Here's how the part is built. I have some questions about the finished solid (model axes, mm). Face numbers are marked on the shaded views. A direction names the side the tool comes from. Give positions to 0.01 mm unless a question says otherwise; leave off trailing zeros. Loops run counter-clockwise (first coordinate to the right, second up) from the corner with the lowest first, then second, coordinate; pieces in that order, holes last. Notation, with made-up numbers: (67.5, -30.5) - (125.5, -30.5) arc R23 cw to (125.5, -11.5) - close; hole circle Ø8 at (63.5, 52). An arc over 180 degrees is marked (long way). Use a Markdown table: item, result.
from build123d import *

# Parameters (mm, degrees)
CUT_EXTRUDE1_DEPTH       = 91
CUT_EXTRUDE13_START      = 79.372539
SKETCH35_W               = 20
SKETCH35_H               = 8.35
CUT_EXTRUDE13_DEPTH      = 10.627461
CIRPATTERN1_COUNT        = 2
CUT_EXTRUDE14_DEPTH      = 64
SKETCH38_W               = 301.896550135
SKETCH38_H               = 232.512752758
CUT_EXTRUDE15_DEPTH      = 13
SKETCH39_W               = 54.010562882
SKETCH39_H               = 10
SKETCH39_W_2             = 56.106077308
BOSS_EXTRUDE1_DEPTH      = 10
SKETCH17_R               = 5.5
CUT_EXTRUDE18_DEPTH      = 181
CUT_EXTRUDE18_DEPTH_BACK = 1
SKETCH42_R               = 15.875
CUT_EXTRUDE19_DEPTH      = 40


with BuildPart() as part:
    # Sketch3 → Revolve2 (revolve)
    with BuildSketch(Plane(origin=(0, 0, 0), x_dir=(0, 0, -1), z_dir=(1, 0, 0))):
        Polygon((-45, 80), (0, 80), (0, 90), (-63, 90), (-63, 15), (-45, 15), (-45, 27.5), (-47.5, 27.5), (-47.5, 73), (-45, 73), align=None)
    revolve(axis=Axis((0, 0, 0), (0, 0, 1)))

    # Sketch4 → Cut-Extrude1 (cut, through all)
    with BuildSketch(Plane(origin=(0, 0, 0), x_dir=(1, 0, 0), z_dir=(0, 1, 0))):
        Polygon((10, -53), (10, -45), (-10, -45), (-10, -53), (-6, -53), (-6, -60), (-10, -60), (-10, -63), (10, -63), (10, -60), (6, -60), (6, -53), align=None)
    cut_extrude1 = extrude(amount=CUT_EXTRUDE1_DEPTH, mode=Mode.SUBTRACT)

    # Sketch35 → Cut-Extrude13 (cut)
    with BuildSketch(Plane(origin=(0, 0, 0), x_dir=(1, 0, 0), z_dir=(0, 1, 0)).offset(CUT_EXTRUDE13_START)):
        with Locations((0, -40.825)):
            Rectangle(SKETCH35_W, SKETCH35_H)
    cut_extrude13 = extrude(amount=CUT_EXTRUDE13_DEPTH, mode=Mode.SUBTRACT)

    # CirPattern1: Cut-Extrude1, Cut-Extrude13 ×2 about axis
    cirpattern1_axis = Axis((0, 0, 0), (0, 0, 1))
    for i in range(1, CIRPATTERN1_COUNT):
        add(cut_extrude1.rotate(cirpattern1_axis, i * 360 / CIRPATTERN1_COUNT), mode=Mode.SUBTRACT)
        add(cut_extrude13.rotate(cirpattern1_axis, i * 360 / CIRPATTERN1_COUNT), mode=Mode.SUBTRACT)

    # Sketch37 → Cut-Extrude14 (cut, through all)
    with BuildSketch(Plane.XY.offset(63)):
        with BuildLine():
            Line((-28, -66.332495807), (-28, -17.464249197))
            ThreePointArc((-28, -17.464249197), (-33, 0), (-28, 17.464249197))
            Line((-28, 17.464249197), (-28, 66.332495807))
            ThreePointArc((-28, 66.332495807), (-72, 0), (-28, -66.332495807))
        make_face()
        with BuildLine():
            Line((28, -17.464249197), (28, -66.332495807))
            ThreePointArc((28, -66.332495807), (72, 0), (28, 66.332495807))
            Line((28, 66.332495807), (28, 17.464249197))
            ThreePointArc((28, 17.464249197), (33, 0), (28, -17.464249197))
        make_face()
    extrude(amount=-CUT_EXTRUDE14_DEPTH, mode=Mode.SUBTRACT)

    # Sketch38 → Cut-Extrude15 (cut)
    with BuildSketch(Plane(origin=(0, 0, 0), x_dir=(-1, 0, 0), z_dir=(0, 0, -1))):
        with Locations((8.285843347, -5.180042081)):
            Rectangle(SKETCH38_W, SKETCH38_H)
    extrude(amount=-CUT_EXTRUDE15_DEPTH, mode=Mode.SUBTRACT)

    # Sketch39 → Boss-Extrude1 (add)
    with BuildSketch(Plane.XY.offset(63)):
        with Locations((47.183112068, 0)):
            Rectangle(SKETCH39_W, SKETCH39_H)
        with Locations((-51.507331201, 0)):
            Rectangle(SKETCH39_W_2, SKETCH39_H)
    extrude(amount=-BOSS_EXTRUDE1_DEPTH)

    # Sketch17 → Cut-Extrude18 (cut, two sides)
    with BuildSketch(Plane(origin=(-90, 0, 0), x_dir=(0, 0, -1), z_dir=(1, 0, 0))) as cut_extrude18_sk:
        with Locations((-27.5, 0)):
            Circle(SKETCH17_R)
    extrude(amount=CUT_EXTRUDE18_DEPTH, mode=Mode.SUBTRACT)
    extrude(cut_extrude18_sk.sketch, amount=-CUT_EXTRUDE18_DEPTH_BACK, mode=Mode.SUBTRACT)

    # Sketch42 → Cut-Extrude19 (cut)
    with BuildSketch(Plane.XY.offset(63)):
        Circle(SKETCH42_R)
    extrude(amount=-CUT_EXTRUDE19_DEPTH, mode=Mode.SUBTRACT)


solid = part.part
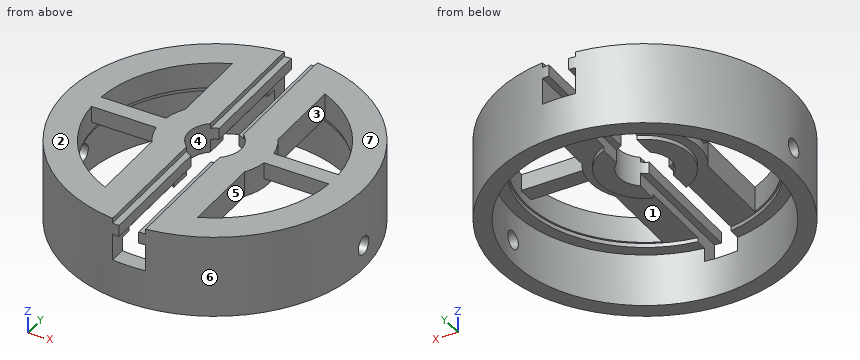
(1) Suppose I cut it at B-B on y = -50.5. Count the separate pieces of the cut face and the enclosed holes in it, plus the area to 3 significant figures.
A:
| item | result |
|---|---|
| separate pieces | 4 |
| enclosed holes | 0 |
| area | 2,240 mm2 |
(2) Suppose I cut it at D-D on x = 50.5. Write out the boundary of the cut face in (y, z).
A:
| item | result |
|---|---|
| outline | (-74.5, 13) - (-62.05, 13) - (-62.05, 45) - (-52.71, 45) - (-52.71, 47.5) - (-51.32, 47.5) - (-51.32, 63) - (-74.5, 63) - close; (-5, 53) - (5, 53) - (5, 63) - (-5, 63) - close; (51.32, 47.5) - (52.71, 47.5) - (52.71, 45) - (62.05, 45) - (62.05, 13) - (74.5, 13) - (74.5, 63) - (51.32, 63) - close |
(3) We'd pull the mould along X, two halves only. Please class the marked faces 4, 5, 6 and 7: pulls with the +X half, pulls with the -X half, needs draft (parallel to the pull), parting line crosses it, or undercut.
A:
| item | result |
|---|---|
| face 4 | undercut |
| face 5 | undercut |
| face 6 | parting line crosses it |
| face 7 | needs draft |
(4) Will these pins go through, and if not, where does the flat tip stop? pin 1 (5 mm diameter, centred on x = -43, z = 57, fed in from -Y); pin 2 (6 mm diameter, centred on x = -57, y = -34, fed in from -Z); pin 3 (4 mm diameter, centred on x = -30.5, z = 45, fed in from -Y); pin 4 (1.2 mm diameter, centred on x = -8, y = -68.5, fed in from +Z).
A:
| item | result |
|---|---|
| pin 1 | y = -80.37 |
| pin 2 | through |
| pin 3 | y = -85.37 |
| pin 4 | z = 60 |
(5) If I drill on line 1 (Z direction, x = 85, y = 0); line 2 (Y direction, x = -41, z = 55); line 3 (X direction, y = 0, z = 34), over which ranges is the centre line in solid material (lowest first)?
A:
| item | result |
|---|---|
| line 1 | 13 to 22, 33 to 63 |
| line 2 | -80.12 to -59.19, -5 to 5, 59.19 to 80.12 |
| line 3 | -90 to -80, 80 to 90 |
(6) On a 3-axis mill with a long thin cutter (end or side, diameter ignored), from which of +Z, -Z, +X, -X, +Y, -Y can I reach the whole of each face in a straight line? I mean the marked faces 1, 2 and 3. Say none if no direction works.
A:
| item | result |
|---|---|
| face 1 | -Z |
| face 2 | +Z, +X, -X, +Y, -Y |
| face 3 | +Z, -Z |
(7) Suppose I cut it at A-A on x = 0. Write out the boundary of the cut face in (y, z), plus the area to 3 significant figures.
A:
| item | result |
|---|---|
| outline | (-90, 13) - (-80, 13) - (-80, 36.65) - (-90, 36.65) - close; (80, 13) - (90, 13) - (90, 36.65) - (80, 36.65) - close |
| area | 473 mm2 |
(8) Suppose I cut it at C-C on z = 27.5. Write out the boundary of the cut face in (x, y).
A:
| item | result |
|---|---|
| outline | (-89.83, -5.5) arc R90 ccw to (89.83, -5.5) - (79.81, -5.5) arc R80 cw to (-79.81, -5.5) - close; (-89.83, 5.5) - (-79.81, 5.5) arc R80 cw to (79.81, 5.5) - (89.83, 5.5) arc R90 ccw to start |
